The model under review builds one solid part; all positions refer to its coordinate system, in mm. Face numbers are marked on the shaded views. A direction names the side the tool comes from. Give positions to 0.01 mm unless a question says otherwise; leave off trailing zeros. Loops run counter-clockwise (first coordinate to the right, second up) from the corner with the lowest first, then second, coordinate; pieces in that order, holes last. Notation, with made-up numbers: (-37, 61) -> (-13, 61) arc R19 ccw to (-13, 89) -> close; hole circle Ø2 at (13.25, 7.5). An arc over 180 degrees is marked (long way). Write each question's results on one line, items separated by ' | '. Start each with the question number.
Q1. Insertion check: pin 1 Ø1 at (x, z) = (-6.5, 19.5) entering from -Y; pin 2 Ø8.5 at (x, z) = (-2, 33) entering from +Y; pin 3 Ø14.5 at (x, y) = (37.5, -10.5) entering from +Z. Each pin has a flat end and moves straight along its axis. Give the tip position at first contact, or say it passes through.
Q2. We need section C-C (x = -15). Write out the cut boundary in (y, z).
Q3. Mouldability with a two-part tool opening along X and no side actions: class the marked faces 6, 7 and 8 as released by +X, released by -X, zero draft, split by the parting line, or undercut.
Q4. We need section A-A (x = 25). Write out the cut boundary in (y, z).
Q5. We need section D-D (y = -69.5). Write out the cut boundary in (x, z), plus the area to 3 significant figures.
Q6. Wall thickness on L1, parallel to X at y = 12.5, z = 8; L2, parallel to Z at x = 0, y = 40.75; L3, parallel to X at y = 45, z = 21: over which ranges is each line inside the solid? List them lowest first. Write a range as [from, to].
Q7. Machinability: for the marked faces 1, 2, 3, 4 and 5, which of the approach directions +Z, -Z, +X, -X, +Y, -Y give a long, thin tool a straight path to every point of the face, cutting with its end or side? Answer none if there is none.
from build123d import *

# Parameters (mm, degrees)
SKETCH_W             = 65
SKETCH_H             = 83
PAD_DEPTH            = 45
SKETCH001_W          = 83
SKETCH001_H          = 32
PAD001_DEPTH         = 15
PAD002_DEPTH         = 15
POCKET_DEPTH         = 403.6691065481
POCKET001_DEPTH      = 500
POCKET001_DEPTH_BACK = 100
PAD003_DEPTH         = 16
SKETCH007_W          = 3
SKETCH007_H          = 135.5960614908
PAD004_DEPTH         = 16
POCKET002_DEPTH      = 414.7315387876
POCKET003_DEPTH      = 5
SKETCH008_W          = 54
SKETCH008_H          = 76
POCKET004_DEPTH      = 35
PAD005_DEPTH         = 65
CHAMFER_SIZE         = 5.3
CHAMFER001_SIZE      = 5.3
CHAMFER002_SIZE      = 0.8999
CHAMFER003_SIZE      = 0.899
CHAMFER004_SIZE      = 0.8999
CHAMFER005_SIZE      = 0.8999
POCKET005_DEPTH      = 80.0010001
POCKET006_DEPTH      = 80.0010001
POCKET007_DEPTH      = 10000
POCKET007_DEPTH_BACK = 100
POCKET008_DEPTH      = 95.001
SKETCH012_W          = 5.5
SKETCH012_H          = 12
POCKET009_DEPTH      = 5
POCKET010_DEPTH      = 20
POCKET010_DEPTH_BACK = 20
POCKET011_DEPTH      = 6
SKETCH014_R          = 8.518625
PAD006_DEPTH         = 13
SKETCH015_R          = 3.5
POCKET012_DEPTH      = 15
SKETCH016_R          = 0.75
POCKET013_DEPTH      = 40
SKETCH018_W          = 5.5
SKETCH018_H          = 12
POCKET014_DEPTH      = 5
POCKET014_FACE131_W  = 12
POCKET014_FACE131_H  = 5.5
PAD007_DEPTH         = 5
POCKET015_DEPTH      = 38.88
POCKET015_DEPTH_BACK = 37
SKETCH020_R          = 3
POCKET016_DEPTH      = 173.1015589479
SKETCH021_R          = 0.75
POCKET017_DEPTH      = 30


with BuildPart() as part:
    # Sketch → Pad (new body)
    with BuildSketch(Plane.XY):
        Rectangle(SKETCH_W, SKETCH_H)
    extrude(amount=PAD_DEPTH)

    # Sketch001 (on Face4 of Pad) → Pad001 (join)
    with BuildSketch(Plane(origin=(-32.5, 0, 0), x_dir=(0, -1, 0), z_dir=(-1, 0, 0))):
        with Locations((0, 29)):
            Rectangle(SKETCH001_W, SKETCH001_H)
    pad001 = extrude(amount=PAD001_DEPTH)

    # Mirrored: Pad001 across YZ
    add(pad001.mirror(Plane.YZ))

    # Sketch002 (on Face4 of Mirrored) → Pad002 (join)
    with BuildSketch(Plane.XZ.offset(41.5)):
        Polygon((-47.5, 45), (47.5, 45), (47.5, 13), (32.5, 13), (32.5, 0), (-32.5, 0), (-32.5, 13), (-47.5, 13), align=None)
    pad002 = extrude(amount=PAD002_DEPTH)

    # Mirrored001: Pad002 across XZ
    add(pad002.mirror(Plane.XZ))

    # Sketch003 (on Face13 of Mirrored001) → Pocket (cut, through all)
    with BuildSketch(Plane(origin=(-47.5, 0, 0), x_dir=(0, -1, 0), z_dir=(-1, 0, 0))):
        Polygon((41.5, 45), (56.5, 0), (69.973511, 50.863071), align=None)
    pocket = extrude(amount=-POCKET_DEPTH, mode=Mode.SUBTRACT)

    # Mirrored002: Pocket across XZ
    add(pocket.mirror(Plane.XZ), mode=Mode.SUBTRACT)

    # Sketch004 → Pocket001 (cut, two sides)
    with BuildSketch(Plane.XZ) as pocket001_sk:
        Polygon((-32.5, 45), (-47.5, 0), (-68.972275, 31.059837), (-58.790833, 51.045628), align=None)
    pocket001 = extrude(amount=-POCKET001_DEPTH, mode=Mode.SUBTRACT) + extrude(pocket001_sk.sketch, amount=POCKET001_DEPTH_BACK, mode=Mode.SUBTRACT)

    # Mirrored003: Pocket001 across YZ
    add(pocket001.mirror(Plane.YZ), mode=Mode.SUBTRACT)

    # Sketch006 (on DatumPlane) → Pad003 (join)
    with BuildSketch(Plane(origin=(-47.5, 0, 4), x_dir=(0, -1, 0), z_dir=(-1, 0, 0))):
        Polygon((-68.401131891, -2.9951612268), (-52.1666666667, 12), (52.1666666667, 12), (67.1949295998, -1.7895363668), (65.1666666666, -4), (52.1666666667, 9), (-52.1666666667, 9), (-66.3655953138, -5.1989286472), align=None)
    pad003 = extrude(amount=-PAD003_DEPTH)

    # Sketch007 (on Face8 of Pad003) → Pad004 (join)
    with BuildSketch(Plane(origin=(0, 0, 0), x_dir=(1, 0, 0), z_dir=(0, 0, -1))):
        with Locations((-31, -0.6031011456)):
            Rectangle(SKETCH007_W, SKETCH007_H)
    pad004 = extrude(amount=-PAD004_DEPTH)

    # Pad004 Face41 → Pocket002 (cut, through all)
    with BuildSketch(Plane(origin=(-32.5, 62.9896434829, 11.0016129244), x_dir=(0, 1, 0), z_dir=(-1, 0, 0))):
        Polygon((5.4114884081, -4.9983870756), (5.4114884081, 9.9967741512), (-10.8229768162, -4.9983870756), align=None)
    pocket002 = extrude(amount=-POCKET002_DEPTH, mode=Mode.SUBTRACT)

    # Pocket002 Face27 → Pocket003 (cut)
    with BuildSketch(Plane(origin=(-32.5, -62.1855086221, 11.4034878777), x_dir=(0, 1, 0), z_dir=(-1, 0, 0))):
        Polygon((10.0188419554, -4.5965121223), (-5.0094209777, 9.1930242445), (-5.0094209777, -4.5965121223), align=None)
    pocket003 = extrude(amount=-POCKET003_DEPTH, mode=Mode.SUBTRACT)

    # Mirrored004: Pad003 across YZ
    add(pad003.mirror(Plane.YZ))

    # Mirrored005: Pad004 across YZ
    add(pad004.mirror(Plane.YZ))

    # Mirrored006: Pocket002 across YZ
    add(pocket002.mirror(Plane.YZ), mode=Mode.SUBTRACT)

    # Mirrored007: Pocket003 across YZ
    add(pocket003.mirror(Plane.YZ), mode=Mode.SUBTRACT)

    # Sketch008 (on Face8 of Mirrored007) → Pocket004 (cut)
    with BuildSketch(Plane(origin=(0, 0, 0), x_dir=(1, 0, 0), z_dir=(0, 0, -1))):
        with Locations((0, -0.8994410524)):
            Rectangle(SKETCH008_W, SKETCH008_H)
    extrude(amount=-POCKET004_DEPTH, mode=Mode.SUBTRACT)

    # Sketch009 (on Face24 of Pocket004) → Pad005 (join)
    with BuildSketch(Plane(origin=(0, -37.1005589476, 0), x_dir=(-1, 0, 0), z_dir=(0, 1, 0))):
        Polygon((-4.7576784019, 45), (-9.5153568039, 36.7594592818), (-4.7576784019, 28.5189185635), (4.7576784019, 28.5189185635), (9.5153568039, 36.7594592818), (4.7576784019, 45), align=None)
    extrude(amount=-PAD005_DEPTH)

    # Chamfer
    chamfer_edges = [part.edges().sort_by_distance(p)[0] for p in [
        (42.166667, 0, 16),
    ]]
    chamfer(chamfer_edges, length=CHAMFER_SIZE)

    # Chamfer001
    chamfer001_edges = [part.edges().sort_by_distance(p)[0] for p in [
        (-42.166667, 0, 16),
    ]]
    chamfer(chamfer001_edges, length=CHAMFER001_SIZE)

    # Chamfer002
    chamfer002_edges = [part.edges().sort_by_distance(p)[0] for p in [
        (-44.816667, -51.166667, 16),
        (-37.333333, -51.166667, 16),
        (-32, -51.166667, 16),
        (-30.5, -51.166667, 16),
    ]]
    chamfer(chamfer002_edges, length=CHAMFER002_SIZE)

    # Chamfer003
    chamfer003_edges = [part.edges().sort_by_distance(p)[0] for p in [
        (30.5, -51.166667, 16),
        (32, -51.166667, 16),
        (37.333333, -51.166667, 16),
        (44.816667, -51.166667, 16),
    ]]
    chamfer(chamfer003_edges, length=CHAMFER003_SIZE)

    # Chamfer004
    chamfer004_edges = [part.edges().sort_by_distance(p)[0] for p in [
        (-30.5, 51.166667, 16),
        (-32, 51.166667, 16),
        (-37.333333, 51.166667, 16),
        (-44.816667, 51.166667, 16),
    ]]
    chamfer(chamfer004_edges, length=CHAMFER004_SIZE)

    # Chamfer005
    chamfer005_edges = [part.edges().sort_by_distance(p)[0] for p in [
        (44.816667, 51.166667, 16),
        (37.333333, 51.166667, 16),
        (32, 51.166667, 16),
        (30.5, 51.166667, 16),
    ]]
    chamfer(chamfer005_edges, length=CHAMFER005_SIZE)

    # Chamfer005 Face72 → Pocket005 (cut, through all)
    with BuildSketch(Plane(origin=(-32.5, 68.0917547069, 0.3349462577), x_dir=(0, 1, 0), z_dir=(-1, 0, 0))):
        Polygon((0.3093771841, 0.3349462577), (-0.6187543683, 0.3349462577), (0.3093771841, -0.6698925155), align=None)
    extrude(amount=-POCKET005_DEPTH, mode=Mode.SUBTRACT)

    # Pocket005 Face105 → Pocket006 (cut, through all)
    with BuildSketch(Plane(origin=(-32.5, -66.5188419554, 0.7368212111), x_dir=(0, 1, 0), z_dir=(-1, 0, 0))):
        Polygon((-0.6760876444, -1.4736424221), (1.3521752888, 0.7368212111), (-0.6760876444, 0.7368212111), align=None)
    extrude(amount=-POCKET006_DEPTH, mode=Mode.SUBTRACT)

    # Pocket006 Face73 → Pocket007 (cut, two sides)
    with BuildSketch(Plane(origin=(-31.5, 66.3350874397, -0.3996428824), x_dir=(0, -1, 0), z_dir=(1, 0, 0))) as pocket007_sk:
        Polygon((1.168420773, -0.3996428824), (-0.0305078741, 0.7992857648), (-1.1379128989, -0.3996428824), align=None)
    extrude(amount=-POCKET007_DEPTH, mode=Mode.SUBTRACT)
    extrude(pocket007_sk.sketch, amount=POCKET007_DEPTH_BACK, mode=Mode.SUBTRACT)

    # Sketch011 (on Face39 of Pocket007) → Pocket008 (cut, through all)
    with BuildSketch(Plane.YZ.offset(47.5)):
        Polygon((65.1666666667, 0), (68.818161, 3.6514943333), (70.985268, 1.013342), (68.517616, -0.789946), align=None)
    extrude(amount=-POCKET008_DEPTH, mode=Mode.SUBTRACT)

    # Sketch012 (on Face30 of Pocket008) → Pocket009 (cut)
    with BuildSketch(Plane(origin=(0, 0, 0), x_dir=(1, 0, 0), z_dir=(0, 0, -1))):
        with Locations((-29.75, -11.8994410524)):
            Rectangle(SKETCH012_W, SKETCH012_H)
    extrude(amount=-POCKET009_DEPTH, mode=Mode.SUBTRACT)

    # Sketch013 → Pocket010 (cut, two sides)
    with BuildSketch(Plane.YZ) as pocket010_sk:
        Polygon((-37.1005589476, 35), (-41.46302, 35), (-53.607724, 0), (-37.1005589476, 0), align=None)
    pocket010 = extrude(amount=-POCKET010_DEPTH, mode=Mode.SUBTRACT) + extrude(pocket010_sk.sketch, amount=POCKET010_DEPTH_BACK, mode=Mode.SUBTRACT)

    # Mirrored008: Pocket010 across XZ
    add(pocket010.mirror(Plane.XZ), mode=Mode.SUBTRACT)

    # Mirrored008 Face101 → Pocket011 (cut)
    with BuildSketch(Plane(origin=(0, 0.2373498677, 35), x_dir=(0, -1, 0), z_dir=(0, 0, -1))):
        Polygon((37.3379088153, 27), (-38.6620911847, 27), (-38.6620911847, 20), (-36.86320908, 20), (-36.86320908, -20), (-38.6620911847, -20), (-38.6620911847, -27), (37.3379088153, -27), (37.3379088153, -20), (37.3379088153, -8.4995325139), (37.3379088153, 8.4995325139), (37.3379088153, 20), align=None)
    extrude(amount=-POCKET011_DEPTH, mode=Mode.SUBTRACT)

    # Sketch014 (on Face128 of Pocket011) → Pad006 (join)
    with BuildSketch(Plane.XZ.offset(-37.1005589476)):
        with Locations((0, 36.4884)):
            Circle(SKETCH014_R)
    extrude(amount=-PAD006_DEPTH)

    # Sketch015 (on Face43 of Pad006) → Pocket012 (cut)
    with BuildSketch(Plane(origin=(0, 50.1005589476, 0), x_dir=(-1, 0, 0), z_dir=(0, 1, 0))):
        with Locations((0, 36.4884)):
            Circle(SKETCH015_R)
    extrude(amount=-POCKET012_DEPTH, mode=Mode.SUBTRACT)

    # Sketch016 (on Face67 of Pocket012) → Pocket013 (cut)
    with BuildSketch(Plane.XZ.offset(102.1005589476)):
        with Locations((0, 57.966855919)):
            Circle(SKETCH016_R)
    extrude(amount=-POCKET013_DEPTH, mode=Mode.SUBTRACT)

    # Sketch018 → Pocket014 (cut)
    with BuildSketch(Plane(origin=(0, 0, 0), x_dir=(1, 0, 0), z_dir=(0, 0, -1))):
        with Locations((29.75, -11.8994410524)):
            Rectangle(SKETCH018_W, SKETCH018_H)
    extrude(amount=-POCKET014_DEPTH, mode=Mode.SUBTRACT)

    # Pocket014 Face131 → Pad007 (add)
    with BuildSketch(Plane(origin=(-29.75, 11.8994410524, 5), x_dir=(0, -1, 0), z_dir=(0, 0, -1))):
        Rectangle(POCKET014_FACE131_W, POCKET014_FACE131_H)
    extrude(amount=PAD007_DEPTH)

    # Sketch019 → Pocket015 (cut, two sides)
    with BuildSketch(Plane.XZ) as pocket015_sk:
        Polygon((-29.5, 16.8537200999), (-36.0278850321, 23.381605132), (-32.1550867428, 35), (-27, 35), (-23.389076, 18.833223), align=None)
    pocket015 = extrude(amount=-POCKET015_DEPTH, mode=Mode.SUBTRACT) + extrude(pocket015_sk.sketch, amount=POCKET015_DEPTH_BACK, mode=Mode.SUBTRACT)

    # Mirrored009: Pocket015 across YZ
    add(pocket015.mirror(Plane.YZ), mode=Mode.SUBTRACT)

    # Sketch020 (on DatumPlane) → Pocket016 (cut, through all)
    with BuildSketch(Plane(origin=(0, 71, 34), x_dir=(1, 0, 0), z_dir=(0, 1, 0))):
        with Locations((-15, 26.885509115)):
            Circle(SKETCH020_R)
        with Locations((15, 26.885509115)):
            Circle(SKETCH020_R)
    extrude(amount=-POCKET016_DEPTH, mode=Mode.SUBTRACT)

    # Sketch021 (on Face71 of Pocket016) → Pocket017 (cut)
    with BuildSketch(Plane.XZ.offset(102.1005589476)):
        with Locations((0, 36.7594592818)):
            Circle(SKETCH021_R)
    extrude(amount=-POCKET017_DEPTH, mode=Mode.SUBTRACT)


solid = part.part
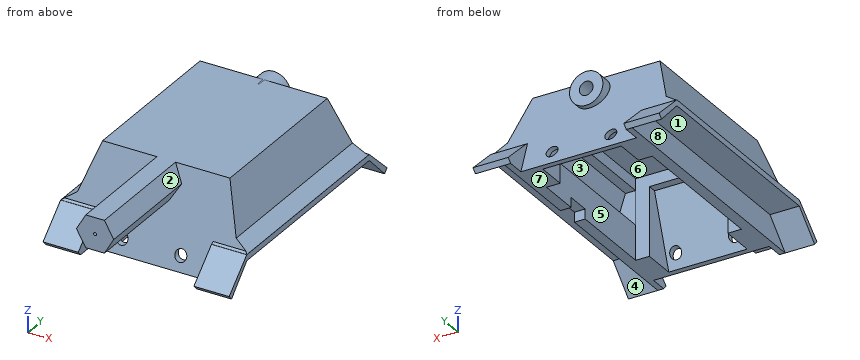
Output:
1) pin 1: y = -50.17 | pin 2: y = 50.1 | pin 3: z = 45
2) outline: (-56.5, 0) -> (-53.61, 0) -> (-52.18, 4.11) -> (-55.13, 4.11) -> close; (-53.13, 10.11) -> (-50.1, 10.11) -> (-41.46, 35) -> (-37.1, 35) -> (-37.1, 41) -> (37.1, 41) -> (37.1, 35) -> (41.46, 35) -> (50.1, 10.11) -> (53.13, 10.11) -> (41.5, 45) -> (-41.5, 45) -> close; (52.18, 4.11) -> (53.61, 0) -> (56.5, 0) -> (55.13, 4.11) -> close
3) face 6: undercut | face 7: zero draft | face 8: released by -X
4) outline: (-56.5, 0) -> (-37.1, 0) -> (-37.1, 41) -> (38.9, 41) -> (38.9, 0) -> (56.5, 0) -> (41.5, 45) -> (-41.5, 45) -> close
5) outline: (-9.52, 36.76) -> (-4.76, 28.52) -> (4.76, 28.52) -> (9.52, 36.76) -> (4.76, 45) -> (-4.76, 45) -> close | area: 235 mm2
6) L1: [-32.5, -27], [27, 32.5] | L2: [27.97, 32.99], [39.99, 45.01] | L3: [-40.53, -20], [20, 40.53]
7) face 1: -Z, -X | face 2: +Z, +X, -Y | face 3: none | face 4: -Z, +X | face 5: -Z
